Read the model definition and answer for the solid it produces. Units are mm, in the model's axes. Round coordinates to 2 decimals unless told otherwise and drop trailing zeros. Write each loop counter-clockwise with the first axis right and the second up, starting at its lowest first coordinate (ties: lowest second). Pieces come first, ordered by that corner, then holes.
from build123d import *

# Parameters (mm, degrees)
F1_DEPTH = 25.4
F2_R     = 12.7
F3_SIZE  = 12.69999


# Not quite as in the source:
# - a fillet or chamfer is up to 0.001 mm smaller than in the source, because OpenCascade refuses the exact size


with BuildPart() as f1:
    # F0 (on Top) → F1 (new body)
    with BuildSketch(Plane.XY):
        with BuildLine():
            ThreePointArc((-50, -30), (-44.1421356237, -44.1421356237), (-30, -50))
            Line((-30, -50), (30, -50))
            ThreePointArc((30, -50), (44.1421356237, -44.1421356237), (50, -30))
            Line((50, -30), (50, 30))
            ThreePointArc((50, 30), (44.1421356237, 44.1421356237), (30, 50))
            Line((30, 50), (-30, 50))
            ThreePointArc((-30, 50), (-44.1421356237, 44.1421356237), (-50, 30))
            Line((-50, 30), (-50, -30))
        make_face()
    extrude(amount=F1_DEPTH)

    # F2
    f2_edges = [f1.edges().sort_by_distance(p)[0] for p in [
        (-44.142136, -44.142136, 0),
        (0, -50, 0),
        (44.142136, -44.142136, 0),
        (50, 0, 0),
        (44.142136, 44.142136, 0),
        (0, 50, 0),
        (-44.142136, 44.142136, 0),
        (-50, 0, 0),
    ]]
    fillet(f2_edges, radius=F2_R)

    # F3 (size 12.7 in the source; OpenCascade refuses exactly that, so slightly less here)
    f3_edges = [f1.edges().sort_by_distance(p)[0] for p in [
        (-44.142136, -44.142136, 25.4),
        (0, -50, 25.4),
        (44.142136, -44.142136, 25.4),
        (50, 0, 25.4),
        (44.142136, 44.142136, 25.4),
        (0, 50, 25.4),
        (-44.142136, 44.142136, 25.4),
        (-50, 0, 25.4),
    ]]
    chamfer(f3_edges, length=F3_SIZE)


solid = f1.part
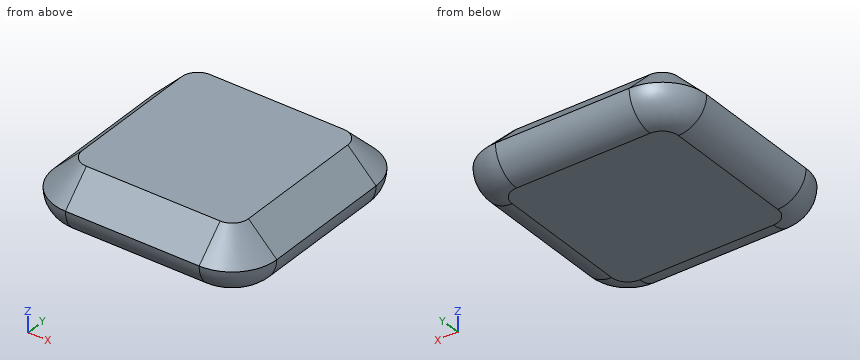
Q1. Straight lines are drawn through the part: probe 1 along Y at (x, z) = (22, 12.5); probe 2 along Z at (x, y) = (0.5, 41.5); probe 3 along X at (y, z) = (-19, 9). For each, find the intervals that lie inside material, in ascending order.
Verdict:
probe 1: y = -50 to 50
probe 2: z = 0.71 to 21.2
probe 3: x = -49.45 to 49.45
Q2. Section A-A (z = 22.5) is taken. Determine the outline of the cut face in (x, y), then the cut area to 3 significant figures.
Verdict:
outline: (-40.2, -30) arc R10.2 ccw to (-30, -40.2) - (30, -40.2) arc R10.2 ccw to (40.2, -30) - (40.2, 30) arc R10.2 ccw to (30, 40.2) - (-30, 40.2) arc R10.2 ccw to (-40.2, 30) - close
area: 6,370 mm2
Q3. Flat-ended cylindrical pins translate along their axes: pin 1 Ø2 at (x, z) = (6.5, 11.5) entering from -Y; pin 2 Ø1 at (x, z) = (2, 11.5) entering from +Y; pin 3 Ø1 at (y, z) = (1, 15.5) entering from +X. Find the tip coordinate at first contact, or state that the pin passes through.
Verdict:
pin 1: stops at y = -50
pin 2: stops at y = 49.98
pin 3: stops at x = 47.7
